```python
from build123d import *

# Parameters (mm, degrees)
BOSS_EXTRUDE1_DEPTH            = 25
SKETCH2_W                      = 2.35
SKETCH2_H                      = 24
CUT_EXTRUDE1_DEPTH             = 23
SKETCH3_R                      = 1.25
CUT_EXTRUDE2_DEPTH             = 58.509648628
CUT_EXTRUDE3_DEPTH             = 58.509648628
CUT_EXTRUDE5_START             = -22
CUT_EXTRUDE5_DEPTH             = 19
CUT_EXTRUDE6_REACH             = 67.815
CUT_EXTRUDE6_END_RADIUS        = 13.5
SKETCH9_W                      = 2.7
SKETCH9_H                      = 13
CUT_EXTRUDE7_REACH             = 67.138
SKETCH10_W                     = 2.7
SKETCH10_H                     = 13
CUT_EXTRUDE7_DIRECTION_2_REACH = 67.138
CUT_EXTRUDE8_DEPTH             = 1.5


with BuildPart() as part:
    # Sketch1 → Boss-Extrude1 (new body)
    with BuildSketch(Plane.XY):
        with BuildLine():
            Line((40, 2.101809534), (40, 32.101809534))
            add(Edge.make_bspline(
                [(40, 32.101809534), (34.329847466, 33.163229144), (26.982496241, 32.840779877), (18.572888448, 31.653354862), (14.859267804, 29.312585721), (9.310772029, 26.484528724)],
                knots=[0, 0, 0, 0, 0.184099436, 0.268179873, 0.840804373, 0.840804373, 0.840804373, 0.840804373], degree=3))
            ThreePointArc((9.310772029, 26.484528724), (2.965735487, 23.839790418), (-3.708097079, 22.192341383))
            ThreePointArc((-3.708097079, 22.192341383), (-22.422953431, -1.860419158), (0, -22.5))
            add(Edge.make_bspline(
                [(40, 2.101809534), (14.753998058, -11.692085759), (19.320151725, -21.091052748), (0, -22.5)],
                knots=[0, 0, 0, 0, 1, 1, 1, 1], degree=3))
        make_face()
    extrude(amount=BOSS_EXTRUDE1_DEPTH)

    # Sketch2 → Cut-Extrude1 (cut)
    with BuildSketch(Plane(origin=(40, 0, 0), x_dir=(0, 0, -1), z_dir=(1, 0, 0))):
        with Locations((-18.675, 16.101809534)):
            Rectangle(SKETCH2_W, SKETCH2_H)
        with Locations((-6.325, 16.101809534)):
            Rectangle(SKETCH2_W, SKETCH2_H)
    extrude(amount=-CUT_EXTRUDE1_DEPTH, mode=Mode.SUBTRACT)

    # Sketch3 → Cut-Extrude2 (cut, through all)
    with BuildSketch(Plane.XY.offset(25)):
        with Locations((30, 21.601809534)):
            Circle(SKETCH3_R)
        with Locations((32, 7.745403073)):
            Circle(SKETCH3_R)
    extrude(amount=-CUT_EXTRUDE2_DEPTH, mode=Mode.SUBTRACT)

    # Sketch4 → Cut-Extrude3 (cut, through all)
    with BuildSketch(Plane.XY.offset(25)):
        with BuildLine():
            Line((10.671834965, 14.77707476), (12.04378968, 15.735776262))
            ThreePointArc((12.04378968, 15.735776262), (21.791242729, 14.007436293), (20.062902761, 4.259983244))
            Line((20.062902761, 4.259983244), (16.966325256, 2.096141048))
            ThreePointArc((16.966325256, 2.096141048), (14.507836146, -0.357822313), (13.037129907, -3.504745895))
            ThreePointArc((13.037129907, -3.504745895), (-11.522414618, -7.034483732), (2.840111071, 13.19786987))
            ThreePointArc((2.840111071, 13.19786987), (6.920533419, 13.171370724), (10.671834965, 14.77707476))
        make_face()
    extrude(amount=-CUT_EXTRUDE3_DEPTH, mode=Mode.SUBTRACT)

    # Sketch6 → Cut-Extrude5 (cut)
    with BuildSketch(Plane.XY.offset(25).offset(CUT_EXTRUDE5_START)):
        with BuildLine():
            Line((-3.708097079, 22.192341383), (-3.378488449, 20.219688816))
            ThreePointArc((-3.378488449, 20.219688816), (-20.432738232, -1.659279471), (-0.071778676, -20.499874337))
            add(Edge.make_bspline(
                [(-0.071778676, -20.499874337), (0.208558967, -20.479056775), (0.777070886, -20.432379755), (1.847267067, -20.326496662), (3.108426982, -20.167703365), (4.494156168, -19.937504643), (6.189724602, -19.579509646), (8.047092499, -19.040626432), (9.948281947, -18.257182138), (11.622649285, -17.334955593), (13.684671017, -15.901647803), (15.442310851, -14.323635678), (16.949424963, -12.863739279), (17.392469361, -12.430339701), (17.53347875, -12.292192277)],
                knots=[0.001319104, 0.001319104, 0.001319104, 0.001319104, 0.016708897, 0.03209869, 0.062878276, 0.093657862, 0.124437448, 0.185996621, 0.247555793, 0.309114965, 0.370674138, 0.493792482, 0.527315904, 0.542705697, 0.542705697, 0.542705697, 0.542705697], degree=3))
            Line((17.53347875, -12.292192277), (18.933119987, -13.720829532))
            add(Edge.make_bspline(
                [(0, -22.5), (10.485156415, -21.735356299), (13.935091868, -18.617416288), (18.933119987, -13.720829532)],
                knots=[0, 0, 0, 0, 0.542705697, 0.542705697, 0.542705697, 0.542705697], degree=3))
            ThreePointArc((0, -22.5), (-22.422953431, -1.860419158), (-3.708097079, 22.192341383))
        make_face()
    extrude(amount=CUT_EXTRUDE5_DEPTH, mode=Mode.SUBTRACT)

    # Cut-Extrude6: up to this cylinder (the profile starts outside it)
    cut_extrude6_end = Plane(origin=(0, 0, 12.5), z_dir=(0, 0, 1)) * Cylinder(CUT_EXTRUDE6_END_RADIUS, 163.63, mode=Mode.PRIVATE)
    # Sketch9 → Cut-Extrude6 (cut, up to the surface)
    with BuildSketch(Plane(origin=(-3.378488449, 20.219688816, 0), x_dir=(0.9863262836854494, 0.16480431460144024, 0), z_dir=(-0.16480431460144024, 0.9863262836854494, 0)), mode=Mode.PRIVATE) as cut_extrude6_sk1:
        with Locations((-1.35, -12.5)):
            Rectangle(SKETCH9_W, SKETCH9_H)
    cut_extrude6_tool1 = extrude(cut_extrude6_sk1.sketch, amount=-CUT_EXTRUDE6_REACH, mode=Mode.PRIVATE) - cut_extrude6_end
    add(cut_extrude6_tool1.solids().sort_by_distance((-4.710029, 19.997203, 12.5))[0], mode=Mode.SUBTRACT)

    # Sketch10 → Cut-Extrude7 (cut, up to next)
    with BuildSketch(Plane(origin=(14.346322684, -14.643531864, 0), x_dir=(-0.7143186274909935, -0.6998206187441061, 0), z_dir=(0.6998206187441061, -0.7143186274909935, 0)), mode=Mode.PRIVATE) as cut_extrude7_sk1:
        with Locations((-2.57216087, -12.5)):
            Rectangle(SKETCH10_W, SKETCH10_H)
    cut_extrude7_tool1 = extrude(cut_extrude7_sk1.sketch, amount=-CUT_EXTRUDE7_REACH, mode=Mode.PRIVATE) & part.part
    add(cut_extrude7_tool1.solids().sort_by_distance((16.183665, -12.843481, 12.5))[0], mode=Mode.SUBTRACT)

    # Sketch10 → Cut-Extrude7 direction 2 (cut, up to next)
    with BuildSketch(Plane(origin=(14.346322684, -14.643531864, 0), x_dir=(-0.7143186274909935, -0.6998206187441061, 0), z_dir=(0.6998206187441061, -0.7143186274909935, 0)), mode=Mode.PRIVATE) as cut_extrude7_direction_2_sk1:
        with Locations((-2.57216087, -12.5)):
            Rectangle(SKETCH10_W, SKETCH10_H)
    cut_extrude7_direction_2_tool1 = extrude(cut_extrude7_direction_2_sk1.sketch, amount=CUT_EXTRUDE7_DIRECTION_2_REACH, mode=Mode.PRIVATE) & part.part
    add(cut_extrude7_direction_2_tool1.solids().sort_by_distance((16.183665, -12.843481, 12.5))[0], mode=Mode.SUBTRACT)

    # Sketch13 → Cut-Extrude8 (cut)
    with BuildSketch(Plane(origin=(0, 0, 0), x_dir=(-1, 0, 0), z_dir=(0, 0, -1))):
        Polygon((-27.75, 20.302771428), (-27.75, 22.900847639), (-30, 24.199885745), (-32.25, 22.900847639), (-32.25, 20.302771428), (-30, 19.003733322), align=None)
        Polygon((-29.75, 9.044441179), (-32, 10.343479284), (-34.25, 9.044441179), (-34.25, 6.446364967), (-32, 5.147326862), (-29.75, 6.446364967), align=None)
    extrude(amount=-CUT_EXTRUDE8_DEPTH, mode=Mode.SUBTRACT)


solid = part.part
```
Verification items for the finished model (mm, model axes). A direction names the side the tool comes from. Round coordinates to 2 decimals unless told otherwise and drop trailing zeros. Order: outer loops, then holes, each group sorted by start corner. A loop starts at its lowest first (then second) coordinate and runs counter-clockwise, first axis right, second up. Notation, with made-up numbers: (51, 89) - (79, 89) arc R36 ccw to (79, 127) - close; hole circle Ø11 at (-21, -2.5). An arc over 180 degrees is marked (long way). Use CSV: the item, a comma, the result in double quotes. Start each with the question number.
1) Access from +Z, -Z, +X, -X, +Y, -Y to the whole of each face (thin tool, end or side, straight path). Record for faces 3 (the flat face through (-17, -12, 3)), 4 (the flat face through (18.536, 3.193, 12.675)), 5 (the flat face through (27.75, 22, 1)), 6 (the flat face through (29, 16, 17.5)).
2) Thickness scan on L1, parallel to Z at x = 33.5, y = 6.5; L2, parallel to Z at x = 24.5, y = 7; L3, parallel to X at y = 8.5, z = 23. Record the ranges inside material, lowest first.
3) Go/stop test with flat-tipped pins: P1, Ø0.8, axis at y = 8, z = 1, coming from the -X side; P2, Ø12.5, axis at x = 4.5, y = -5, coming from the +Z side; P3, Ø12, axis at x = 21.5, z = 8.5, coming from the -Y side; P4, Ø2, axis at x = 7, z = 8.5, coming from the -Y side. Record where each tip stops, or that it passes through.
4) Mould release check, pull along X, two halves, no side actions. Record for faces 1 (the flat face through (30, 4.102, 6)), 2 (the cylindrical face through (30.672, 22.656, 3.351)): +X half, -X half, draft (parallel to the pull), parting line (faces both ways), or undercut.
5) Section check A-A, the plane x = -8. Record the cut outline in (y, z), plus the area to 3 significant figures.
6) Section check B-B, the plane y = -11.5. State how many separate pieces and enclosed holes the cut face has, plus the area to 3 significant figures.
Answers:
1,face 3,"none"
1,face 4,"+Z, -Z"
1,face 5,"-Z"
1,face 6,"+X"
2,L1,"z = 1.5 to 5.15, 7.5 to 17.5, 19.85 to 25"
2,L2,"z = 0 to 5.15, 7.5 to 17.5, 19.85 to 25"
2,L3,"x = -20.83 to -10.49, 22.89 to 31, 33 to 40"
3,P1,"stops at x = -21.18"
3,P2,"passes through"
3,P3,"stops at y = -14.24"
3,P4,"stops at y = -19.6"
4,face 1,"draft"
4,face 2,"undercut"
5,outline,"(-21.03, 0) - (-10.87, 0) - (-10.87, 25) - (-21.03, 25) - (-21.03, 22) - (-18.87, 22) - (-18.87, 3) - (-21.03, 3) - close; (10.87, 0) - (21.03, 0) - (21.03, 3) - (18.87, 3) - (18.87, 22) - (21.03, 22) - (21.03, 25) - (10.87, 25) - close"
5,area,"426 mm²"
6,separate pieces,"2"
6,enclosed holes,"1"
6,area,"566 mm²"
